from build123d import *

# Parameters (mm, degrees)
EXTRUDE_1_DEPTH      = 16
EXTRUDE_2_DEPTH      = 12
EXTRUDE_3_DEPTH      = 12
EXTRUDE_3_DEPTH_BACK = 35
FILLET_1_R           = 1
EXTRUDE_4_DEPTH      = 4
EXTRUDE_4_DEPTH_BACK = 12
FILLET_2_R           = 2
SKETCH_5_R           = 1.5
CUT_EXTRUDE_1_DEPTH  = 0.1
SKETCH_6_R           = 1
CUT_EXTRUDE_2_DEPTH  = 0.1


with BuildPart() as part:
    # ｽｹｯﾁ1 → ﾎﾞｽ - 押し出し1 (new body)
    with BuildSketch(Plane.XY):
        with BuildLine():
            Line((5, 0), (17, 0))
            ThreePointArc((17, 0), (20.535533906, 1.464466094), (22, 5))
            Line((22, 5), (22, 24.8))
            ThreePointArc((22, 24.8), (20.535533906, 28.335533906), (17, 29.8))
            Line((17, 29.8), (5, 29.8))
            ThreePointArc((5, 29.8), (1.464466094, 28.335533906), (0, 24.8))
            Line((0, 24.8), (0, 5))
            ThreePointArc((0, 5), (1.464466094, 1.464466094), (5, 0))
        make_face()
    extrude(amount=EXTRUDE_1_DEPTH)

    # ｽｹｯﾁ2 → ﾎﾞｽ - 押し出し2 (add)
    with BuildSketch(Plane.XY.offset(16)):
        with BuildLine():
            Line((17, 27.8), (5, 27.8))
            ThreePointArc((5, 27.8), (2.878679656, 26.921320344), (2, 24.8))
            Line((2, 24.8), (2, 5))
            ThreePointArc((2, 5), (2.878679656, 2.878679656), (5, 2))
            Line((5, 2), (17, 2))
            ThreePointArc((17, 2), (19.121320344, 2.878679656), (20, 5))
            Line((20, 5), (20, 24.8))
            ThreePointArc((20, 24.8), (19.121320344, 26.921320344), (17, 27.8))
        make_face()
    extrude(amount=EXTRUDE_2_DEPTH)

    # ｽｹｯﾁ3 → ﾎﾞｽ - 押し出し3 (add, two sides: drawn at the far end of the back side and taken through both)
    with BuildSketch(Plane.XY.offset(28).offset(-EXTRUDE_3_DEPTH_BACK)):
        with BuildLine():
            ThreePointArc((4.341687605, 12.4), (3, 14.9), (4.341687605, 17.4))
            ThreePointArc((4.341687605, 17.4), (3.878679656, 22.021320344), (8.5, 21.558312395))
            ThreePointArc((8.5, 21.558312395), (13.121320344, 22.021320344), (12.658312395, 17.4))
            ThreePointArc((12.658312395, 17.4), (14, 14.9), (12.658312395, 12.4))
            ThreePointArc((12.658312395, 12.4), (13.121320344, 7.778679656), (8.5, 8.241687605))
            ThreePointArc((8.5, 8.241687605), (3.878679656, 7.778679656), (4.341687605, 12.4))
        make_face()
    extrude(amount=EXTRUDE_3_DEPTH + EXTRUDE_3_DEPTH_BACK)

    # ﾌｨﾚｯﾄ1
    fillet_1_edges = [part.edges().sort_by_distance(p)[0] for p in [
        (1.464466094, 28.335533906, 16),
        (11, 29.8, 0),
        (20.535533906, 28.335533906, 0),
        (0, 14.9, 16),
        (1.464466094, 1.464466094, 16),
        (11, 0, 16),
        (20.535533906, 1.464466094, 16),
        (22, 14.9, 16),
        (19.121320344, 26.921320344, 28),
        (11, 27.8, 28),
        (2.878679656, 26.921320344, 28),
        (2, 14.9, 28),
        (2.878679656, 2.878679656, 28),
        (11, 2, 28),
        (19.121320344, 2.878679656, 28),
        (20, 14.9, 28),
        (20.535533906, 28.335533906, 16),
        (11, 29.8, 16),
        (22, 14.9, 0),
        (20.535533906, 1.464466094, 0),
        (11, 0, 0),
        (1.464466094, 1.464466094, 0),
        (0, 14.9, 0),
        (1.464466094, 28.335533906, 0),
    ]]
    fillet(fillet_1_edges, radius=FILLET_1_R - 0.0001)  # a hair under: the kernel refuses the full size

    # ｽｹｯﾁ4 → ﾎﾞｽ - 押し出し4 (add, two sides: drawn at the far end of the back side and taken through both)
    with BuildSketch(Plane(origin=(20, 0, 0), x_dir=(0, 0, -1), z_dir=(1, 0, 0)).offset(-EXTRUDE_4_DEPTH_BACK)):
        Polygon((-27, 20.9), (-40, 20.9), (-40, 8.9), (-27, 8.9), (-18.970751541, 8.9), (-18.970751541, 20.9), align=None)
    extrude(amount=EXTRUDE_4_DEPTH + EXTRUDE_4_DEPTH_BACK)

    # ﾌｨﾚｯﾄ2
    fillet_2_edges = [part.edges().sort_by_distance(p)[0] for p in [
        (24, 8.9, 29.48537577),
        (24, 20.9, 29.48537577),
    ]]
    fillet(fillet_2_edges, radius=FILLET_2_R)

    # ｽｹｯﾁ5 → ｶｯﾄ - 押し出し1 (cut)
    with BuildSketch(Plane(origin=(0, 0, -7), x_dir=(-1, 0, 0), z_dir=(0, 0, -1))):
        with Locations((-11, 19.9)):
            Circle(SKETCH_5_R)
        with Locations((-11, 14.9)):
            Circle(SKETCH_5_R)
        with Locations((-11, 9.9)):
            Circle(SKETCH_5_R)
        with Locations((-6, 19.9)):
            Circle(SKETCH_5_R)
        with Locations((-6, 14.9)):
            Circle(SKETCH_5_R)
        with Locations((-6, 9.9)):
            Circle(SKETCH_5_R)
    extrude(amount=-CUT_EXTRUDE_1_DEPTH, mode=Mode.SUBTRACT)

    # ｽｹｯﾁ6 → ｶｯﾄ - 押し出し2 (cut)
    with BuildSketch(Plane.XY.offset(40)):
        with Locations((11, 19.9)):
            Circle(SKETCH_6_R)
        with Locations((11, 14.811145862)):
            Circle(SKETCH_6_R)
        with Locations((11, 9.9)):
            Circle(SKETCH_6_R)
        with Locations((6, 19.9)):
            Circle(SKETCH_6_R)
        with Locations((6, 14.9)):
            Circle(SKETCH_6_R)
        with Locations((6, 9.9)):
            Circle(SKETCH_6_R)
    extrude(amount=-CUT_EXTRUDE_2_DEPTH, mode=Mode.SUBTRACT)


solid = part.part
Could you check a few things on this model? Use its own coordinates, in mm. A direction names the side the tool comes from. Give positions to 0.01 mm unless a question says otherwise; leave off trailing zeros. Order: outer loops, then holes, each group sorted by start corner. A loop starts at its lowest first (then second) coordinate and runs counter-clockwise, first axis right, second up. Notation, with made-up numbers: (33.5, 72) -> (58.5, 72) arc R27 ccw to (58.5, 111) -> close; hole circle Ø4 at (89, 12). An arc over 180 degrees is marked (long way). Return JSON: item names as keys, results as strings.
1. Thinking about a two-plate mould opening in Y: for faces 4 (the cylindrical face through (2.9, 26.94, 21.42)), 5 (the flat face through (6, 15, -6.9)), 6 (the flat face through (24, 15, 30)), which applies, pulls with the +Y half, pulls with the -Y half, needs draft (parallel to the pull), parting line crosses it, or undercut?
Answer list:
{"face 4": "pulls with the +Y half", "face 5": "undercut", "face 6": "needs draft"}
2. Imagine slicing it at A-A on y = 23.75. List the corners of the cut face in (x, z) for me, then the cut area to 3 significant figures.
Answer list:
{"outline": "(0, 1) arc R1 ccw to (1, 0) -> (21, 0) arc R1 ccw to (22, 1) -> (22, 15) arc R1 ccw to (21, 16) -> (20, 16) -> (20, 27) arc R1 ccw to (19, 28) -> (3, 28) arc R1 ccw to (2, 27) -> (2, 16) -> (1, 16) arc R1 ccw to (0, 15) -> close", "area": "567 mm2"}
3. Imagine slicing it at C-C on z = 13. List the corners of the cut face in (x, y) for me.
Answer list:
{"outline": "(0, 5) arc R5 ccw to (5, 0) -> (17, 0) arc R5 ccw to (22, 5) -> (22, 24.8) arc R5 ccw to (17, 29.8) -> (5, 29.8) arc R5 ccw to (0, 24.8) -> close"}
4. For pin 1 Ø8 at (y, z) = (11.5, 22.5) entering from -X; pin 2 Ø2.5 at (x, z) = (19, 29) entering from -Y; pin 3 Ø9 at (x, z) = (10.5, 21.5) entering from -Y, each with a flat end and sliding along its axis, tell me the tip position at first contact or that it passes through.
Answer list:
{"pin 1": "stops at x = 2", "pin 2": "stops at y = 2.97", "pin 3": "stops at y = 2"}
5. On a 3-axis mill with a long thin cutter (end or side, diameter ignored), from which of +Z, -Z, +X, -X, +Y, -Y can I reach the whole of each face in a straight line? I mean faces 1 (the flat face through (6, 10, -6.9)), 2 (the cylindrical face through (19.715, 22.877, 27.699)), 3 (the cylindrical face through (2.86, 2.9, 21.42)). Say none if no direction works.
Answer list:
{"face 1": "-Z", "face 2": "+Z, +X, +Y", "face 3": "+Z, -X, -Y"}
6. I need wall thicknesses on line 1 (X direction, y = 13.5, z = 2); line 2 (Z direction, x = 15.5, y = 9.5); line 3 (Z direction, x = 18.25, y = 6.25). Which ranges of each line are inside material? Lowest first, please. Write a range as from..to.
Answer list:
{"line 1": "x = 0..22", "line 2": "z = 0..40", "line 3": "z = 0..28"}
7. Imagine slicing it at B-B on z = 25. List the corners of the cut face in (x, y) for me, then the cut area to 3 significant figures.
Answer list:
{"outline": "(2, 5) arc R3 ccw to (5, 2) -> (17, 2) arc R3 ccw to (20, 5) -> (20, 8.9) -> (22, 8.9) arc R2 ccw to (24, 10.9) -> (24, 18.9) arc R2 ccw to (22, 20.9) -> (20, 20.9) -> (20, 24.8) arc R3 ccw to (17, 27.8) -> (5, 27.8) arc R3 ccw to (2, 24.8) -> close", "area": "503 mm2"}
